Check sheet for the modelled part. Datum: model origin and axes. Units: mm. Face numbers are marked on the shaded views. A direction names the side the tool comes from. Coordinates: 2 decimals unless noted, no trailing zeros. Write each loop counter-clockwise with the first axis right and the second up, starting at its lowest first coordinate (ties: lowest second). Pieces come first, ordered by that corner, then holes. Notation, with made-up numbers: (49, 10) - (95, 10) arc R26 cw to (95, 45) - close; hole circle Ø7 at (-1.75, -26.75). An arc over 180 degrees is marked (long way). Write each question's results on one line, items separated by ' | '.
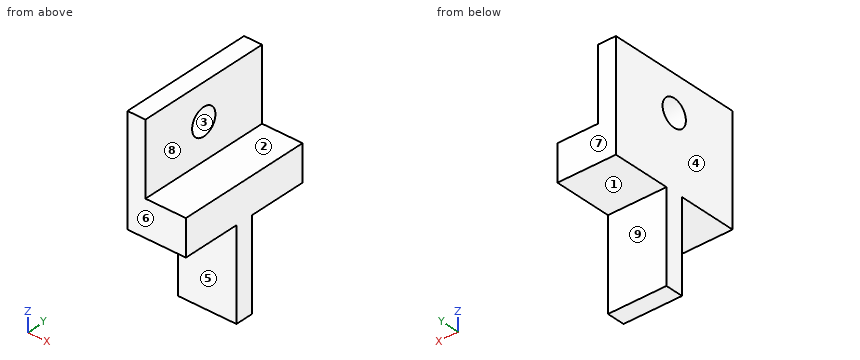
from build123d import *

# Parameters (mm, degrees)
SKETCH1_W           = 30
SKETCH1_H           = 15
BOSS_EXTRUDE1_DEPTH = 2
SKETCH2_W           = 6.5
SKETCH2_H           = 15
BOSS_EXTRUDE2_DEPTH = 4
SKETCH3_W           = 6.5
SKETCH3_H           = 2
BOSS_EXTRUDE3_DEPTH = 10
SKETCH4_R           = 2
CUT_EXTRUDE2_DEPTH  = 5
BOSS_EXTRUDE4_START = 5
SKETCH5_R           = 3.5
SKETCH5_R_2         = 2
BOSS_EXTRUDE4_DEPTH = 5
SKETCH6_W           = 22
SKETCH6_H           = 15
CUT_EXTRUDE3_DEPTH  = 10
SKETCH7_R           = 1.5
CUT_EXTRUDE4_DEPTH  = 10


with BuildPart() as part:
    # Sketch1 → Boss-Extrude1 (new body)
    with BuildSketch(Plane(origin=(0, 0, 0), x_dir=(0, 0, -1), z_dir=(1, 0, 0))):
        with Locations((15, 7.5)):
            Rectangle(SKETCH1_W, SKETCH1_H)
    extrude(amount=BOSS_EXTRUDE1_DEPTH)

    # Sketch2 → Boss-Extrude2 (add)
    with BuildSketch(Plane(origin=(0, 0, -30), x_dir=(-1, 0, 0), z_dir=(0, 0, -1))):
        with Locations((-3.25, 7.5)):
            Rectangle(SKETCH2_W, SKETCH2_H)
    extrude(amount=BOSS_EXTRUDE2_DEPTH)

    # Sketch3 → Boss-Extrude3 (add)
    with BuildSketch(Plane(origin=(0, 0, -34), x_dir=(-1, 0, 0), z_dir=(0, 0, -1))):
        with Locations((-3.25, 7.5)):
            Rectangle(SKETCH3_W, SKETCH3_H)
    extrude(amount=BOSS_EXTRUDE3_DEPTH)

    # Sketch4 → Cut-Extrude2 (cut)
    with BuildSketch(Plane(origin=(2, 0, 0), x_dir=(0, 0, -1), z_dir=(1, 0, 0))):
        with Locations((10, 7.5)):
            Circle(SKETCH4_R)
    extrude(amount=-CUT_EXTRUDE2_DEPTH, mode=Mode.SUBTRACT)

    # Sketch5 → Boss-Extrude4 (add)
    with BuildSketch(Plane(origin=(2, 0, 0), x_dir=(0, 0, -1), z_dir=(1, 0, 0)).offset(BOSS_EXTRUDE4_START)):
        with Locations(Location((10, 7.5, 0), (0, 0, 180))):
            Circle(SKETCH5_R)
        with Locations((10, 7.5)):
            Circle(SKETCH5_R_2, mode=Mode.SUBTRACT)
    extrude(amount=-BOSS_EXTRUDE4_DEPTH)

    # Sketch6 → Cut-Extrude3 (cut)
    with BuildSketch(Plane.ZY):
        with Locations((-11, 7.5)):
            Rectangle(SKETCH6_W, SKETCH6_H)
    extrude(amount=-CUT_EXTRUDE3_DEPTH, mode=Mode.SUBTRACT)

    # Sketch7 → Cut-Extrude4 (cut)
    with BuildSketch(Plane.ZY):
        with Locations((-26, 7.5)):
            Circle(SKETCH7_R)
    extrude(amount=-CUT_EXTRUDE4_DEPTH, mode=Mode.SUBTRACT)


solid = part.part
1. Sectioned sample at D-D (x = 3.75). Record the cut outline in (y, z), then the cut area to 3 significant figures.
Values follow:
outline: (0, -34) - (6.5, -34) - (6.5, -44) - (8.5, -44) - (8.5, -34) - (15, -34) - (15, -30) - (0, -30) - close | area: 80.0 mm^2
2. Draft check along Z on the marked faces 1, 2, 3 and 4. Enter one of: pulls with the +Z half, pulls with the -Z half, needs draft (parallel to the pull), parting line crosses it, or undercut.
Values follow:
face 1: pulls with the -Z half | face 2: pulls with the +Z half | face 3: undercut | face 4: needs draft
3. Sectioned sample at B-B (z = -26). Record the cut outline in (x, y), then the cut area to 3 significant figures.
Values follow:
outline: (0, 0) - (2, 0) - (2, 6) - (0, 6) - close; (0, 9) - (2, 9) - (2, 15) - (0, 15) - close | area: 24.0 mm^2
4. Sectioned sample at A-A (y = 7.5). Record the cut outline in (x, z).
Values follow:
outline: (0, -44) - (6.5, -44) - (6.5, -30) - (2, -30) - (2, -27.5) - (0, -27.5) - close; (0, -24.5) - (2, -24.5) - (2, -22) - (0, -22) - close
5. Sectioned sample at C-C (x = 1). Record the cut outline in (y, z).
Values follow:
outline: (0, -34) - (6.5, -34) - (6.5, -44) - (8.5, -44) - (8.5, -34) - (15, -34) - (15, -22) - (0, -22) - close; hole circle Ø3 at (7.5, -26)
6. Material ranges on L1, parallel to Y at x = 0.6, z = -26; L2, parallel to Z at x = 1.25, y = 1.25; L3, parallel to X at y = 13, z = -27.75, recorded low to high. Write a range as [from, to].
Values follow:
L1: y = [0, 6], [9, 15] | L2: z = [-34, -22] | L3: x = [0, 2]
7. Access from +Z, -Z, +X, -X, +Y, -Y to the whole of each face (thin tool, end or side, straight path). Record for the marked faces 5, 6, 7, 8 and 9.
Values follow:
face 5: -Z, +X, -X, -Y | face 6: +Z, -Z, +X, -X, -Y | face 7: +Z, -Z, +X, -X, +Y | face 8: +Z, +X, +Y, -Y | face 9: -Z, +X, -X, +Y
8. Go/stop test with flat-tipped pins: pin 1 (3 mm diameter, centred on y = 10.5, z = -37.5, fed in from -X); pin 2 (1.5 mm diameter, centred on x = 1.5, z = -37, fed in from -Y); pin 3 (2 mm diameter, centred on x = 4.5, y = 9, fed in from +Z); pin 4 (9 mm diameter, centred on y = 7, z = -27.5, fed in from +X). Record where each tip stops, or that it passes through.
Values follow:
pin 1: passes through | pin 2: stops at y = 6.5 | pin 3: stops at z = -30 | pin 4: stops at x = 6.5
